Source: CAD feature listing. Evaluate the final solid. Frame: model axes, mm. A direction names the side the tool comes from. Give positions to 0.01 mm unless a question says otherwise; leave off trailing zeros. Write each loop counter-clockwise with the first axis right and the second up, starting at its lowest first coordinate (ties: lowest second). Pieces come first, ordered by that corner, then holes. Notation, with made-up numbers: (76, 15.5) -> (127, 15.5) arc R24 cw to (127, 44.5) -> close; hole circle Ø6 at (77, -11). An arc over 180 degrees is marked (long way). Answer as a JSON object with one key per item and string values. Group by question number.
Item 1: First-contact query: pin 1 Ø1.5 at (y, z) = (-8.5, 24) entering from -X; pin 2 Ø1.5 at (x, y) = (43.5, -9) entering from +Z; pin 3 Ø1.5 at (y, z) = (-7, 27) entering from -X; pin 4 Ø1 at (y, z) = (-5.5, 20) entering from -X. Flat tips, straight axial feed; report the tip coordinate or a pass-through.
Item 2: Section query A-A on x = 42. Return the cut outline in (y, z).
Item 3: Section query C-C on z = 30.5. Return the cut outline in (x, y), plus the area to 3 significant figures.
Item 4: Section query D-D on x = 45. Return the cut outline in (y, z).
Item 5: Section query B-B on y = -7. Return the cut outline in (x, z), plus the area to 3 significant figures.
Item 6: Access query for faces 1 (the face through (43.474, -8.352, 25.818)), 2 (the face through (43.474, -8.352, 8.479)), 3 (the face through (42, -7, 39)). Directions: +Z, -Z, +X, -X, +Y, -Y. A direction counts if a zero-diameter tool reaches every point of the face in a straight line with its end or side. Return the directions, or none.
Item 7: Ray query, probe 1 along Z at (x, y) = (45.25, -9.5); probe 2 along X at (y, z) = (-6, 33); probe 3 along Y at (x, z) = (43, 19.5). Return the intervals inside material, ascending. Write a range as from..to.
from build123d import *

# Parameters (mm, degrees)
BOX018_W                  = 15
BOX018_H                  = 6
BOX018_DEPTH              = 3
CYLINDER058_R             = 1.5
CYLINDER058_DEPTH         = 25
CYLINDER057_R             = 2
CYLINDER057_DEPTH         = 32
FUSION041_PLACEMENT_ANGLE = 180


with BuildPart() as cube015:
    # Box018 → Box018 (new body)
    with BuildSketch(Plane(origin=(58.2, 67, 3), x_dir=(1, 0, 0), z_dir=(0, 0, 1))):
        with Locations((7.5, 3)):
            Rectangle(BOX018_W, BOX018_H)
    extrude(amount=BOX018_DEPTH)


with BuildPart() as cylinder058:
    # Cylinder058 → Cylinder058 (new body)
    with BuildSketch(Plane(origin=(70, 70, 7), x_dir=(1, 0, 0), z_dir=(0, 0, 1))):
        Circle(CYLINDER058_R)
    extrude(amount=CYLINDER058_DEPTH)


with BuildPart() as bohrungfanductupper001:
    # Cylinder057 → Cylinder057 (new body)
    with BuildSketch(Plane(origin=(70, 70, 0), x_dir=(1, 0, 0), z_dir=(0, 0, 1))):
        Circle(CYLINDER057_R)
    extrude(amount=CYLINDER057_DEPTH)

    # Fusion041: union Cube015, Cylinder058
    add(cube015.part)
    add(cylinder058.part)


with BuildPart() as bohrungfanductupper001_1:
    # Fusion041 placement: moved
    add(bohrungfanductupper001.part.moved(Location((112, 63, 7))).rotate(Axis((112, 63, 7), (0, 0, 1)), FUSION041_PLACEMENT_ANGLE))


solid = bohrungfanductupper001_1.part
Worked answers:
{
 "1": {"pin 1": "x = 40.15", "pin 2": "z = 39", "pin 3": "x = 40", "pin 4": "x = 40.27"},
 "2": {"outline": "(-10, 10) -> (-9, 10) -> (-9, 7) -> (-5, 7) -> (-5, 10) -> (-4, 10) -> (-4, 13) -> (-5, 13) -> (-5, 39) -> (-9, 39) -> (-9, 13) -> (-10, 13) -> close"},
 "3": {"outline": "circle Ø4 at (42, -7)", "area": "12.6 mm^2"},
 "4": {"outline": "(-10, 10) -> (-4, 10) -> (-4, 13) -> (-10, 13) -> close"},
 "5": {"outline": "(38.8, 10) -> (40, 10) -> (40, 7) -> (44, 7) -> (44, 10) -> (53.8, 10) -> (53.8, 13) -> (44, 13) -> (44, 39) -> (40, 39) -> (40, 13) -> (38.8, 13) -> close", "area": "161 mm^2"},
 "6": {"face 1": "+Z", "face 2": "-Z", "face 3": "+Z, +X, -X, +Y, -Y"},
 "7": {"probe 1": "10..13", "probe 2": "40.27..43.73", "probe 3": "-8.73..-5.27"}
}
